The listing builds one solid part. Answer for the finished solid, in the listing's coordinates (mm). A direction names the side the tool comes from. Coordinates: 2 decimals unless noted, no trailing zeros. Loops run counter-clockwise (first coordinate to the right, second up) from the corner with the lowest first, then second, coordinate; pieces in that order, holes last. Notation, with made-up numbers: M 44,53.5 L 94,53.5 A22 cw 94,65.5 Z; hole C 27.25,56 d5. An arc over 180 degrees is marked long. Answer as a JSON object with one key per item and string values. Group by question number.
1. A cutting plane is placed at A-A on x = 1.5. Give the vertices of the cut face in (y, z).
2. Straight lines are drawn through the part: L1, parallel to X at y = 46.5, z = -0.25; L2, parallel to X at y = 6, z = -2.25; L3, parallel to Z at x = 3, y = 2. For each, find the intervals that lie inside material, in ascending order.
3. A cutting plane is placed at D-D on y = 6.5. Give the vertices of the cut face in (x, z).
4. A cutting plane is placed at C-C on z = 0. Give the vertices of the cut face in (x, y).
5. Given pin 1 (1.5 mm diameter, centred on x = -0.5, z = 0, fed in from +Y); pin 2 (3 mm diameter, centred on x = 2, z = 1.5, fed in from +Y); pin 3 (2 mm diameter, centred on y = 41, z = -3, fed in from -X); pin 4 (1 mm diameter, centred on x = -2, y = 38, fed in from -Z), each flat-ended and moving along its own axis, determine where each tip first touches the part or whether it passes through.
6. Determine the mould class of faces 1 (the face through (0, 11.036, 0)), 2 (the face through (0.9, 26.3, 3.9)), 3 (the face through (-2, 53.34, 2)) for opening direction Z: released by +Z, released by -Z, zero draft, split by the parting line, or undercut.
7. A cutting plane is placed at B-B on y = 35. Give the vertices of the cut face in (x, z).
8. For faces 4 (the face through (-2, 0, 2)), 5 (the face through (1.441, 5.595, 1.736)), 6 (the face through (0, 42.304, 0)), determine the directions among +Z, -Z, +X, -X, +Y, -Y from which every point of the face is accessible in a straight line to the end or side of a thin tool.
Autodesk Inventor part; units mm, degrees
ref_plane "Work Plane1" through (0, 26.67, 0) normal (0, -1, 0) x (1, 0, 0)
ref_plane "YZ Plane" through (0, 0, 0) normal (1, 0, 0) x (0, 1, 0)
ref_plane "XZ Plane" through (0, 0, 0) normal (0, 1, 0) x (-1, 0, 0)
sketch "Sketch1" plane through (0, 0, 0) normal (0, 1, 0) x (-1, 0, 0)
  circle A0 centre (0, 0) radius 4.0005
  dimension "d0" = 8.001
extrude "Extrusion1" add sketch "Sketch1" along normal blind 53.34
ref_plane "Work Plane1" through (0, 26.67, 0) normal (0, -1, 0) x (1, 0, 0)
sketch "Sketch3" plane through (0, 0, 0) normal (0, -1, 0) x (1, 0, 0)
  point P0 (0, 0)
  point P1 (-0.1045, -0.2801)
hole "Hole1" at (-0.1045, 0, -0.2801) direction (0, 1, 0) diameter 5.08 depth 11.0363
sketch "Sketch4" plane through (0, 53.34, 0) normal (0, 1, 0) x (1, 0, 0)
  point P0 (0, 0)
  point P1 (0.1091, 0.0558)
hole "Hole2" at (0.1091, 53.34, -0.0558) direction (0, -1, 0) diameter 5.08 depth 11.0363
properties part number "central rotator claw grabber_3DPrint"
From the geometry:
{
 "1": {"outline": "M 0,-3.71 L 53.34,-3.71 L 53.34,-2.18 L 42.3,-2.18 L 42.3,2.07 L 53.34,2.07 L 53.34,3.71 L 0,3.71 L 0,1.69 L 11.04,1.69 L 11.04,-2.25 L 0,-2.25 Z"},
 "2": {"L1": "x = -3.99 to -2.42, 2.64 to 3.99", "L2": "x = -3.31 to -1.71, 1.5 to 3.31", "L3": "z = -2.65 to 2.65"},
 "3": {"outline": "C 0,0 d8; hole C -0.1,-0.28 d5.08"},
 "4": {"outline": "M -4,0 L -2.63,0 L -2.63,11.04 L 2.42,11.04 L 2.42,0 L 4,0 L 4,53.34 L 2.65,53.34 L 2.65,42.3 L -2.43,42.3 L -2.43,53.34 L -4,53.34 Z"},
 "5": {"pin 1": "stops at y = 42.3", "pin 2": "stops at y = 53.34", "pin 3": "stops at x = -3.46", "pin 4": "stops at z = -3.71"},
 "6": {"face 1": "undercut", "face 2": "split by the parting line", "face 3": "zero draft"},
 "7": {"outline": "C 0,0 d8"},
 "8": {"face 4": "+Z, -Z, +X, -X, -Y", "face 5": "-Y", "face 6": "+Y"}
}
